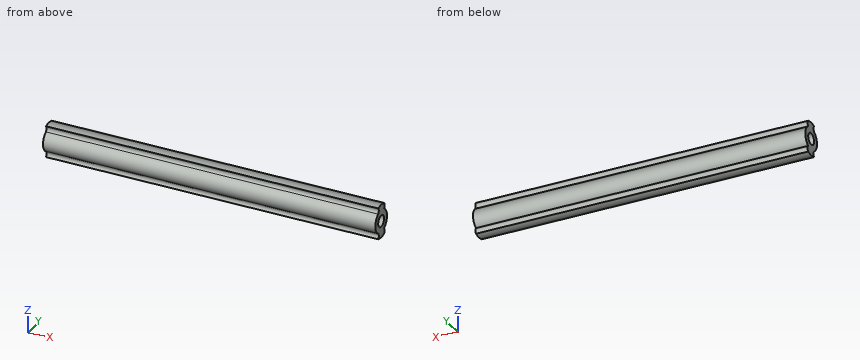
from build123d import *

# Parameters (mm, degrees)
SKETCH1_R           = 10
SKETCH1_R_2         = 5
BOSS_EXTRUDE1_DEPTH = 290


with BuildPart() as part:
    # Sketch1 → Boss-Extrude1 (new body)
    # profile 1 of 3: a face of its own
    with BuildSketch(Plane(origin=(0, 0, 0), x_dir=(0, 0, -1), z_dir=(1, 0, 0))):
        Circle(SKETCH1_R)
        Circle(SKETCH1_R_2, mode=Mode.SUBTRACT)
    # profile 2 of 3: a face of its own
    with BuildSketch(Plane(origin=(0, 0, 0), x_dir=(0, 0, -1), z_dir=(1, 0, 0))):
        with BuildLine():
            ThreePointArc((8.656235338, 5.006954141), (9.658218091, 2.59206931), (10, 0))
            ThreePointArc((10, 0), (9.657587422, -2.594418084), (8.653798961, -5.011163891))
            ThreePointArc((8.653798961, -5.011163891), (11.157678989, -3.972789688), (13.662430885, -5.009059016))
            ThreePointArc((13.662430885, -5.009059016), (14.533959389, -0.004529508), (13.662430885, 5))
            ThreePointArc((13.662430885, 5), (11.160773363, 6.040295531), (8.656235338, 5.006954141))
        make_face()
    # profile 3 of 3: a face of its own
    with BuildSketch(Plane(origin=(0, 0, 0), x_dir=(0, 0, -1), z_dir=(1, 0, 0))):
        with BuildLine():
            ThreePointArc((-8.653798961, -5.011163891), (-9.999999704, -0.002431971), (-8.656235338, 5.006954141))
            ThreePointArc((-8.656235338, 5.006954141), (-11.160773363, 6.040295531), (-13.662430885, 5))
            ThreePointArc((-13.662430885, 5), (-14.533959389, -0.004529508), (-13.662430885, -5.009059016))
            ThreePointArc((-13.662430885, -5.009059016), (-11.157678989, -3.972789688), (-8.653798961, -5.011163891))
        make_face()
    extrude(amount=BOSS_EXTRUDE1_DEPTH)


solid = part.part
For this review, take the finished solid that the model builds, in its own axes (mm). Give positions to 0.01 mm unless a question says otherwise; leave off trailing zeros. Loops run counter-clockwise (first coordinate to the right, second up) from the corner with the lowest first, then second, coordinate; pieces in that order, holes last. Notation, with made-up numbers: M -6.5,21 L 10.5,21 A24 ccw 10.5,48 Z; hole C 77.25,16 d3. An arc over 180 degrees is marked long. Answer as a JSON object with one key per item and string values. Group by question number.
Q1. Insertion check: P1, Ø3, axis at x = 43.5, y = 4, coming from the -Z side; P2, Ø5, axis at x = 65, y = 5, coming from the +Z side; P3, Ø8, axis at x = 240.5, z = -11, coming from the -Y side. Each pin has a flat end and moves straight along its axis. Give the tip position at first contact, or say it passes through.
Q2. Add section A-A on z = 0. Give the boundary of the cut face in (x, y), and give its area (3 significant figures).
Q3. Add section B-B on x = 65.5. Give the boundary of the cut face in (y, z), and give its area (3 significant figures).
Q4. Add section C-C on y = 0. Give the boundary of the cut face in (x, z), and give its area (3 significant figures).
Q5. For probe 1 along Z at (x, y) = (68.5, 0.75); probe 2 along Y at (x, z) = (213, 0.5); probe 3 along Z at (x, y) = (171, 5.25), list the stretches that pass through material, from the lowest coordinate up. Write a range as [from, to].
Checked values:
{
 "1": {"P1": "z = -14.32", "P2": "z = 14.32", "P3": "y = -7.14"},
 "2": {"outline": "M 0,-10 L 290,-10 L 290,-5 L 0,-5 Z; M 0,5 L 290,5 L 290,10 L 0,10 Z", "area": "2,900 mm²"},
 "3": {"outline": "M -5.01,-13.66 A14.8 ccw 5,-13.66 A3.54 ccw 5.01,-8.66 A10 ccw 5.01,8.66 A3.54 ccw 5,13.66 A14.8 ccw -5.01,13.66 A3.54 cw -5.01,8.65 A10 ccw -5.01,-8.65 A3.54 cw Z; hole C 0,0 d10", "area": "329 mm²"},
 "4": {"outline": "M 0,-14.53 L 290,-14.53 L 290,-5 L 0,-5 Z; M 0,5 L 290,5 L 290,14.53 L 0,14.53 Z", "area": "5,530 mm²"},
 "5": {"probe 1": "[-14.51, -4.94], [4.94, 14.51]", "probe 2": "[-9.99, -4.97], [4.97, 9.99]", "probe 3": "[-13.39, -8.93], [-8.51, 8.51], [8.93, 13.39]"}
}
